The model under review builds one solid part; all positions refer to its coordinate system, in mm. Face numbers are marked on the shaded views. A direction names the side the tool comes from. Coordinates: 2 decimals unless noted, no trailing zeros. Order: outer loops, then holes, each group sorted by start corner. A loop starts at its lowest first (then second) coordinate and runs counter-clockwise, first axis right, second up. Notation, with made-up numbers: M 70.5,35.5 L 127.5,35.5 A9 cw 127.5,44.5 Z; hole C 23,31 d8. An arc over 180 degrees is marked long. One line per item, written item: value.
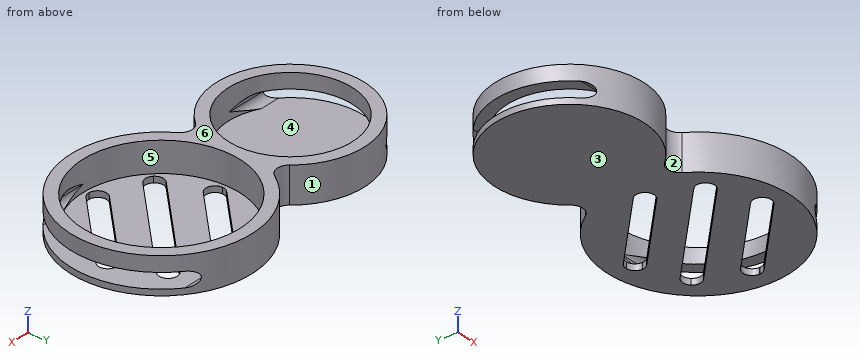
```python
from build123d import *

# Parameters (mm, degrees)
F0_R      = 10.3
F0_R_2    = 13.1
F1_DEPTH  = 1
F2_DEPTH  = 6
F5_DEPTH  = 28.7
F8_DEPTH  = 25.9
F10_DEPTH = 25


with BuildPart() as f1:
    # F0 (on Top) → F1 (new body)
    with BuildSketch(Plane.XY):
        with BuildLine():
            ThreePointArc((-1.864875, -7.891034), (-0.200569, -7.178368), (1.357094, -8.101132))
            ThreePointArc((1.357094, -8.101132), (29.2, 0), (1.357094, 8.101132))
            ThreePointArc((1.357094, 8.101132), (-0.200569, 7.178368), (-1.864875, 7.891034))
            ThreePointArc((-1.864875, 7.891034), (-23.6, 0), (-1.864875, -7.891034))
        make_face()
        with Locations((-11.3, 0)):
            Circle(F0_R, mode=Mode.SUBTRACT)
        with Locations((14.1, 0)):
            Circle(F0_R_2, mode=Mode.SUBTRACT)
        with Locations((-11.3, 0)):
            Circle(F0_R)
        with Locations((14.1, 0)):
            Circle(F0_R_2)
    extrude(amount=F1_DEPTH)

    # F0 (on Top) → F2 (join)
    with BuildSketch(Plane.XY):
        with BuildLine():
            ThreePointArc((-1.864875, -7.891034), (-0.200569, -7.178368), (1.357094, -8.101132))
            ThreePointArc((1.357094, -8.101132), (29.2, 0), (1.357094, 8.101132))
            ThreePointArc((1.357094, 8.101132), (-0.200569, 7.178368), (-1.864875, 7.891034))
            ThreePointArc((-1.864875, 7.891034), (-23.6, 0), (-1.864875, -7.891034))
        make_face()
        with Locations((-11.3, 0)):
            Circle(F0_R, mode=Mode.SUBTRACT)
        with Locations((14.1, 0)):
            Circle(F0_R_2, mode=Mode.SUBTRACT)
    extrude(amount=F2_DEPTH)

    # F4 (on offset) → F5 (cut)
    with BuildSketch(Plane.YZ.offset(-40)):
        with BuildLine():
            ThreePointArc((10.3, 2.25), (9.933883, 3.133883), (9.05, 3.5))
            Line((9.05, 3.5), (-9.05, 3.5))
            ThreePointArc((-9.05, 3.5), (-9.933883, 3.133883), (-10.3, 2.25))
            ThreePointArc((-10.3, 2.25), (-9.933883, 1.366117), (-9.05, 1))
            Line((-9.05, 1), (9.05, 1))
            ThreePointArc((9.05, 1), (9.933883, 1.366117), (10.3, 2.25))
        make_face()
    extrude(amount=F5_DEPTH, mode=Mode.SUBTRACT)

    # F7 (on offset) → F8 (cut)
    with BuildSketch(Plane.YZ.offset(40)):
        with BuildLine():
            Line((11.85, 3.5), (-11.85, 3.5))
            ThreePointArc((-11.85, 3.5), (-12.733883, 3.133883), (-13.1, 2.25))
            ThreePointArc((-13.1, 2.25), (-12.733883, 1.366117), (-11.85, 1))
            Line((-11.85, 1), (11.85, 1))
            ThreePointArc((11.85, 1), (12.733883, 1.366117), (13.1, 2.25))
            ThreePointArc((13.1, 2.25), (12.733883, 3.133883), (11.85, 3.5))
        make_face()
    extrude(amount=-F8_DEPTH, mode=Mode.SUBTRACT)

    # F9 (on face) → F10 (cut)
    with BuildSketch(Plane.XY.offset(1)):
        with BuildLine():
            ThreePointArc((15.547263, 9.932544), (13.425942, 9.932544), (13.425942, 12.053864))
            Line((13.425942, 12.053864), (2.046136, 0.674058))
            ThreePointArc((2.046136, 0.674058), (3.680821, 0.999217), (4.606796, -0.386602))
            ThreePointArc((4.606796, -0.386602), (4.492615, -0.960628), (4.167456, -1.447263))
            Line((4.167456, -1.447263), (15.547263, 9.932544))
        make_face()
        with BuildLine():
            ThreePointArc((15.986602, 10.993204), (15.565741, 12.035059), (14.539321, 12.492277))
            ThreePointArc((14.539321, 12.492277), (13.937023, 12.388898), (13.425942, 12.053864))
            ThreePointArc((13.425942, 12.053864), (13.425942, 9.932544), (15.547263, 9.932544))
            ThreePointArc((15.547263, 9.932544), (15.872422, 10.419179), (15.986602, 10.993204))
        make_face()
        with BuildLine():
            ThreePointArc((2.046136, 0.674058), (1.711102, 0.162977), (1.607723, -0.439321))
            ThreePointArc((1.607723, -0.439321), (2.557216, -1.782297), (4.167456, -1.447263))
            ThreePointArc((4.167456, -1.447263), (4.492615, -0.960628), (4.606796, -0.386602))
            ThreePointArc((4.606796, -0.386602), (3.680821, 0.999217), (2.046136, 0.674058))
        make_face()
        with BuildLine():
            ThreePointArc((22.938835, 6.717514), (23.378175, 7.778175), (22.938835, 8.838835))
            ThreePointArc((22.938835, 8.838835), (21.878175, 9.278175), (20.817514, 8.838835))
            Line((20.817514, 8.838835), (13.03934, 1.06066))
            Line((13.03934, 1.06066), (5.261165, -6.717514))
            ThreePointArc((5.261165, -6.717514), (4.821825, -7.778175), (5.261165, -8.838835))
            ThreePointArc((5.261165, -8.838835), (6.321825, -9.278175), (7.382486, -8.838835))
            Line((7.382486, -8.838835), (22.938835, 6.717514))
        make_face()
        with BuildLine():
            ThreePointArc((26.153864, -0.674058), (24.032544, -0.674058), (24.032544, 1.447263))
            Line((24.032544, 1.447263), (12.652737, -9.932544))
            ThreePointArc((12.652737, -9.932544), (14.287423, -9.607385), (15.213398, -10.993204))
            ThreePointArc((15.213398, -10.993204), (15.099217, -11.567229), (14.774058, -12.053864))
            Line((14.774058, -12.053864), (26.153864, -0.674058))
        make_face()
        with BuildLine():
            ThreePointArc((12.652737, -9.932544), (12.317703, -11.542784), (13.660679, -12.492277))
            ThreePointArc((13.660679, -12.492277), (14.262977, -12.388898), (14.774058, -12.053864))
            ThreePointArc((14.774058, -12.053864), (15.099217, -11.567229), (15.213398, -10.993204))
            ThreePointArc((15.213398, -10.993204), (14.287423, -9.607385), (12.652737, -9.932544))
        make_face()
        with BuildLine():
            ThreePointArc((26.593204, 0.386602), (26.592973, 0.412966), (26.592277, 0.439321))
            ThreePointArc((26.592277, 0.439321), (25.642784, 1.782297), (24.032544, 1.447263))
            ThreePointArc((24.032544, 1.447263), (24.032544, -0.674058), (26.153864, -0.674058))
            ThreePointArc((26.153864, -0.674058), (26.479023, -0.187423), (26.593204, 0.386602))
        make_face()
    extrude(amount=-F10_DEPTH, mode=Mode.SUBTRACT)


solid = f1.part
```
(1) Mouldability with a two-part tool opening along Y and no side actions: class the marked faces 1, 2, 3 and 4 as +Y half, -Y half, draft (parallel to the pull), parting line (faces both ways), or undercut.
Geometry results:
face 1: parting line
face 2: -Y half
face 3: draft
face 4: undercut
(2) We need section B-B, the plane x = 6.5. State the section outline as (y, z) points.
Geometry results:
outline: M -13.05,0 L -9.27,0 L -9.27,1 L -10.67,1 L -10.67,6 L -13.05,6 Z; M -5.48,0 L 0.89,0 L 0.89,1 L -5.48,1 Z; M 5.13,0 L 13.05,0 L 13.05,6 L 10.67,6 L 10.67,1 L 5.13,1 Z
(3) We need section A-A, the plane y = -3. State the section outline as (x, z) points.
Geometry results:
outline: M -23.23,0 L 8.98,0 L 8.98,1 L 1.35,1 L 1.35,6 L -1.45,6 L -1.45,1 L -23.23,1 Z; M -23.23,3.5 L -21.15,3.5 L -21.15,6 L -23.23,6 Z; M 13.22,0 L 19.59,0 L 19.59,1 L 13.22,1 Z; M 23.83,0 L 28.9,0 L 28.9,1 L 23.83,1 Z; M 26.85,3.5 L 28.9,3.5 L 28.9,6 L 26.85,6 Z
(4) We need section D-D, the plane x = -4. State the section outline as (y, z) points.
Geometry results:
outline: M -9.9,0 L 9.9,0 L 9.9,6 L 7.27,6 L 7.27,1 L -7.27,1 L -7.27,6 L -9.9,6 Z
(5) For L1, parallel to Y at x = 14.1, z = 3.2; L2, parallel to Y at x = -11.3, z = 4.5; L3, parallel to X at y = 0, z = 3.3, list the stretches that pass through material, from the lowest coordinate up.
Geometry results:
L1: y = -15.1 to -13.1, 13.1 to 15.1
L2: y = -12.3 to -10.3, 10.3 to 12.3
L3: x = -1 to 1
(6) Insertion check: pin 1 Ø5 at (x, y) = (-2.5, 8.5) entering from -Z; pin 2 Ø3 at (x, y) = (22, 2) entering from +Z; pin 3 Ø1.5 at (y, z) = (-10, 2.5) entering from -X; pin 4 Ø2 at (x, z) = (17.5, 2) entering from +Y. Each pin has a flat end and moves straight along its axis. Give the tip position at first contact, or say it passes through.
Geometry results:
pin 1: stops at z = 0
pin 2: stops at z = 1
pin 3: stops at x = -18.7
pin 4: stops at y = 14.91
(7) Tool access review of the marked faces 5 and 6: name each direction out of +Z, -Z, +X, -X, +Y, -Y from which nothing blocks a thin tool from reaching the whole face with its end or side.
Geometry results:
face 5: +Z
face 6: +Z, +X, -X, +Y, -Y
(8) We need section C-C, the plane z = 3. State the section outline as (x, y) points.
Geometry results:
outline: M -18.39,-10.05 A12.3 ccw -1.86,-7.89 A2 cw 1.36,-8.1 A15.1 ccw 22.03,-12.85 L 16.65,-12.85 A13.1 cw long 16.65,12.85 L 22.03,12.85 A15.1 ccw 1.36,8.1 A2 cw -1.86,7.89 A12.3 ccw -18.39,10.05 L -13.56,10.05 A10.3 cw long -13.56,-10.05 Z
